Geometry: see drawing. Coordinates: mm, zero at the bounding-box minimum. A direction names the side the tool comes from. Give positions to 0.01 mm unless a question says otherwise; leave off trailing zeros. Loops run counter-clockwise (first coordinate to the right, second up) from the corner with the lowest first, then second, coordinate; pieces in that order, holes last. Notation, with made-up numbers: (7, -22) - (22, -22) arc R8 ccw to (22, -7) - close; hole circle Ø2 at (1.25, 69). An arc over 180 degrees is marked (long way). Use one line per item in the form item = value.
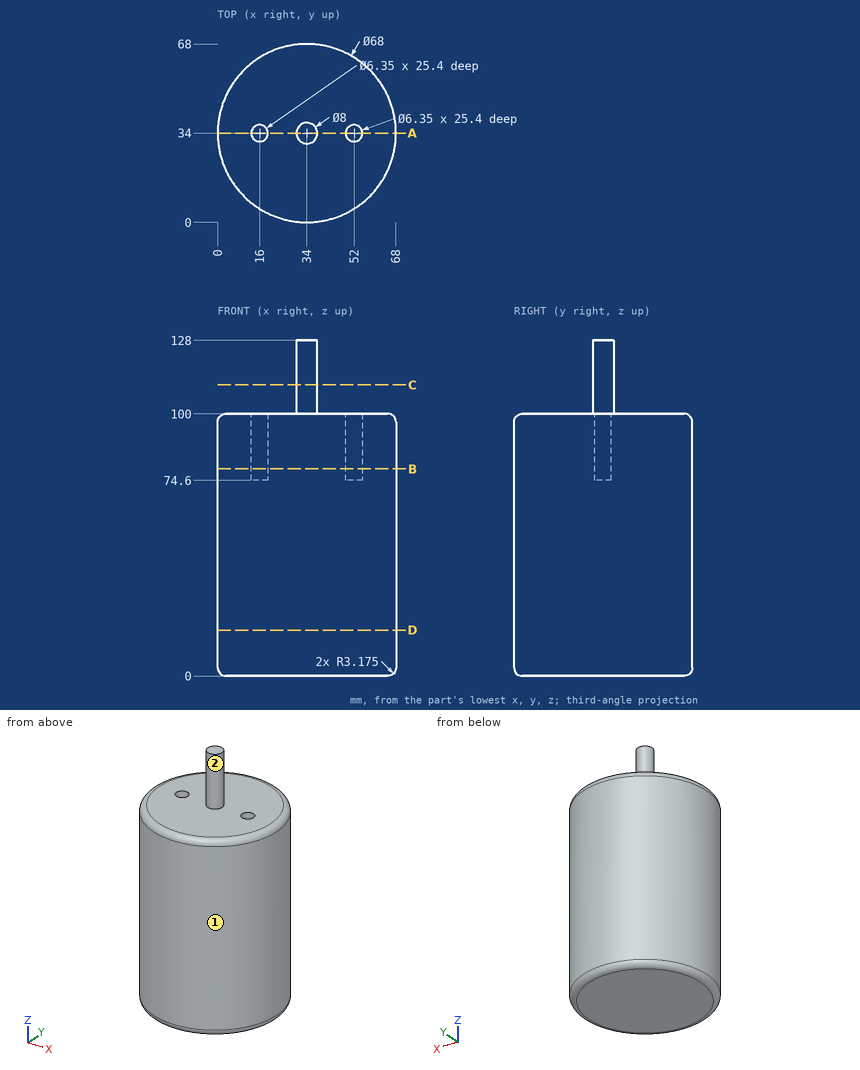
(1) Pin query (flat end, axial travel): P1, Ø3, axis at x = 53.5, y = 36.5, coming from the +Z side; P2, Ø1, axis at y = 25, z = 71.5, coming from the +X side; P3, Ø10, axis at x = 8.5, z = 104, coming from the +Y side. Return the tip coordinate at first contact, or that it passes through.
Solution:
P1 = 100
P2 = 66.92
P3 = 56.69
(2) Cut plane C-C (z = 111). Return the cut outline in (x, y).
Solution:
outline = circle Ø8 at (34, 34)
(3) Access query for the marked faces 1 and 2. Directions: +Z, -Z, +X, -X, +Y, -Y. A direction counts if a zero-diameter tool reaches every point of the face in a straight line with its end or side. Return the directions, or none.
Solution:
face_1 = +Z, -Z
face_2 = +Z
(4) Material intervals for L1, parallel to Z at x = 24, y = 63.5; L2, parallel to Z at x = 17, y = 35.5; L3, parallel to Y at x = 16, z = 90 (3 decimals), sorted ascending. Write a range as from..to.
Solution:
L1 = 0.02..99.98
L2 = 0..74.6
L3 = 5.156..30.825, 37.175..62.844
(5) Cut plane D-D (z = 17.5). Return the cut outline in (x, y).
Solution:
outline = circle Ø68 at (34, 34)
(6) Cut plane A-A (y = 34). Return the cut outline in (x, z) (3 decimals).
Solution:
outline = (0, 3.175) arc R3.175 ccw to (3.175, 0) - (64.825, 0) arc R3.175 ccw to (68, 3.175) - (68, 96.825) arc R3.175 ccw to (64.825, 100) - (55.175, 100) - (55.175, 74.6) - (48.825, 74.6) - (48.825, 100) - (38, 100) - (38, 128) - (30, 128) - (30, 100) - (19.175, 100) - (19.175, 74.6) - (12.825, 74.6) - (12.825, 100) - (3.175, 100) arc R3.175 ccw to (0, 96.825) - close
(7) Cut plane B-B (z = 79). Return the cut outline in (x, y) (3 decimals).
Solution:
outline = circle Ø68 at (34, 34); hole circle Ø6.35 at (16, 34); hole circle Ø6.35 at (52, 34)
